from build123d import *

# Parameters (mm, degrees)
PALM_BODY_DEPTH     = 9
SKETCH7_W           = 18
SKETCH7_H           = 26.918715159
BOSS_EXTRUDE1_DEPTH = 15


with BuildPart() as part:
    # Palm_sketch → Palm_Body (new, symmetric)
    with BuildSketch(Plane.XY):
        with BuildLine():
            Line((-36.5, 78.60257579), (36.5, 78.60257579))
            ThreePointArc((36.5, 78.60257579), (42.156854249, 76.259430039), (44.5, 70.60257579))
            Line((44.5, 70.60257579), (44.5, 3.401763707))
            ThreePointArc((44.5, 3.401763707), (43.86206295, 0.271263888), (42.04999272, -2.359970476))
            Line((42.04999272, -2.359970476), (19.004994037, -24.558074529))
            ThreePointArc((19.004994037, -24.558074529), (18.045809386, -25.179685068), (16.923746767, -25.39742421))
            Line((16.923746767, -25.39742421), (-16.891594266, -25.39742421))
            ThreePointArc((-16.891594266, -25.39742421), (-18.012780844, -25.180038208), (-18.971480575, -24.55938465))
            Line((-18.971480575, -24.55938465), (-42.04636349, -2.360489531))
            ThreePointArc((-42.04636349, -2.360489531), (-43.861076957, 0.27192072), (-44.5, 3.404738308))
            Line((-44.5, 3.404738308), (-44.5, 70.60257579))
            ThreePointArc((-44.5, 70.60257579), (-42.156854249, 76.259430039), (-36.5, 78.60257579))
        make_face()
    extrude(amount=PALM_BODY_DEPTH, both=True)


with BuildPart() as body_2:
    # Sketch7 → Boss-Extrude1 (new body)
    with BuildSketch(Plane.ZY.offset(44.5)):
        with Locations((0, 16.864095887)):
            Rectangle(SKETCH7_W, SKETCH7_H)
    extrude(amount=-BOSS_EXTRUDE1_DEPTH)


with BuildPart() as part_1:
    add(part.part)

    # Combine1: cut body 2
    add(body_2.part, mode=Mode.SUBTRACT)


solid = part_1.part
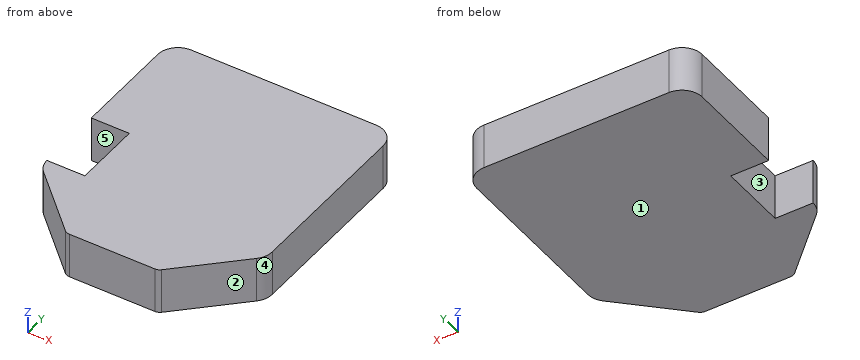
Input: part model. Units: mm. Frame: model coordinates. Face numbers are marked on the shaded views. A direction names the side the tool comes from. Give positions to 0.01 mm unless a question says otherwise; leave off trailing zeros. Write each loop counter-clockwise with the first axis right and the second up, starting at its lowest first coordinate (ties: lowest second). Pieces come first, ordered by that corner, then holes.
Q1. Pull-direction query (X, two-part tool) for the marked faces 1, 2 and 3; classes: pulls with the +X half, pulls with the -X half, needs draft (parallel to the pull), parting line crosses it, or undercut.
Q2. Section B-B, the plane x = -33.5. Output: boundary loops of the cut face in (y, z), plus the area to 3 significant figures.
Q3. Section C-C, the plane y = 7. Output: boundary loops of the cut face in (x, z), plus the area to 3 significant figures.
Q4. Section A-A, the plane z = -6.5. Output: boundary loops of the cut face in (x, y) (3 decimals), plus the area to 3 significant figures.
Q5. Set-up query: the marked faces 4 and 5. Return all of +Z, -Z, +X, -X, +Y, -Y with unobstructed straight access to the full face (end or side cutting, diameter ignored); none if empty.
Q6. First-contact query: P1, Ø4.5, axis at x = -37.5, z = 3, coming from the -Y side; P2, Ø10, axis at y = -3.5, z = -4.5, coming from the +X side; P3, Ø5.5, axis at y = 20.5, z = -2.5, coming from the -X side. Flat tips, straight axial feed; report the tip coordinate or a pass-through.
Q7. Material intervals for probe 1 along X at (y, z) = (19.5, 6.5); probe 2 along Y at (x, z) = (-38, -0.25); probe 3 along Y at (x, z) = (17, -5), sorted ascending.
Q8. Section D-D, the plane x = -23.5. Output: boundary loops of the cut face in (y, z).
Filled in:
1. face 1: needs draft
1. face 2: pulls with the +X half
1. face 3: pulls with the -X half
2. outline: (-10.58, -9) - (3.4, -9) - (3.4, 9) - (-10.58, 9) - close; (30.32, -9) - (78.6, -9) - (78.6, 9) - (30.32, 9) - close
2. area: 1,120 mm2
3. outline: (-29.5, -9) - (44.5, -9) - (44.5, 9) - (-29.5, 9) - close
3. area: 1,330 mm2
4. outline: (-44.5, 3.405) arc R8 ccw to (-42.046, -2.36) - (-18.971, -24.559) arc R3 ccw to (-16.892, -25.397) - (16.924, -25.397) arc R3 ccw to (19.005, -24.558) - (42.05, -2.36) arc R8 ccw to (44.5, 3.402) - (44.5, 70.603) arc R8 ccw to (36.5, 78.603) - (-36.5, 78.603) arc R8 ccw to (-44.5, 70.603) - (-44.5, 30.323) - (-29.5, 30.323) - (-29.5, 3.405) - close
4. area: 8,150 mm2
5. face 4: +Z, -Z, +X, -Y
5. face 5: +Z, -Z, -X
6. P1: stops at y = -8.9
6. P2: stops at x = 44.27
6. P3: stops at x = -29.5
7. probe 1: x = -29.5 to 44.5
7. probe 2: y = -6.25 to 3.4, 30.32 to 78.46
7. probe 3: y = -25.4 to 78.6
8. outline: (-20.2, -9) - (78.6, -9) - (78.6, 9) - (-20.2, 9) - close
